Here's how the part is built. I have some questions about the finished solid (model axes, mm). Face numbers are marked on the shaded views. Round coordinates to 2 decimals unless told otherwise and drop trailing zeros. One line per item, written item: value. Start each with the question number.
Item 1: Thinking about a two-plate mould opening in Z: for the marked faces 1 and 2, which applies, released by +Z, released by -Z, zero draft, split by the parting line, or undercut?
Item 2: If I drill on line 1 (Y direction, x = -150.75, z = 1.25); line 2 (X direction, y = -2.25, z = 0.7); line 3 (X direction, y = 10.5, z = 0.45), over which ranges is the centre line in solid material (lowest first)?
Item 3: For P1, Ø8, axis at x = -150.75, y = 0, coming from the +Z side, with a flat end and sliding along its axis, tell me the tip position at first contact or that it passes through.
```python
from build123d import *

# Parameters (mm, degrees)
BOSS_EXTRUDE1_DEPTH = 3
SKETCH2_R           = 2.5
CUT_EXTRUDE1_DEPTH  = 4


with BuildPart() as part:
    # Sketch1 → Boss-Extrude1 (new body)
    with BuildSketch(Plane.XY):
        with BuildLine():
            Line((155.75, 15), (0, 15))
            Line((0, 15), (0, 0))
            Line((0, 0), (160.75, 0))
            Line((160.75, 0), (160.75, 10))
            ThreePointArc((160.75, 10), (159.285533906, 13.535533906), (155.75, 15))
        make_face()
        with BuildLine():
            Line((0, 15), (-155.75, 15))
            ThreePointArc((-155.75, 15), (-159.285533906, 13.535533906), (-160.75, 10))
            Line((-160.75, 10), (-160.75, 0))
            Line((-160.75, 0), (0, 0))
            Line((0, 0), (0, 15))
        make_face()
        with BuildLine():
            Line((0, -15), (0, 0))
            Line((0, 0), (-160.75, 0))
            Line((-160.75, 0), (-160.75, -10))
            ThreePointArc((-160.75, -10), (-159.285533906, -13.535533906), (-155.75, -15))
            Line((-155.75, -15), (0, -15))
        make_face()
        with BuildLine():
            Line((160.75, 0), (0, 0))
            Line((0, 0), (0, -15))
            Line((0, -15), (155.75, -15))
            ThreePointArc((155.75, -15), (159.285533906, -13.535533906), (160.75, -10))
            Line((160.75, -10), (160.75, 0))
        make_face()
    extrude(amount=BOSS_EXTRUDE1_DEPTH)

    # Sketch2 → Cut-Extrude1 (cut, through all)
    with BuildSketch(Plane(origin=(0, 0, 0), x_dir=(-1, 0, 0), z_dir=(0, 0, -1))):
        with BuildLine():
            ThreePointArc((-153.120541102, 0), (-150.620541102, -2.5), (-148.120541102, 0))
            Line((-148.120541102, 0), (-153.120541102, 0))
        make_face()
        with BuildLine():
            Line((-153.120541102, 0), (-148.120541102, 0))
            ThreePointArc((-148.120541102, 0), (-150.620541102, 2.5), (-153.120541102, 0))
        make_face()
        with Locations((150.75, 0)):
            Circle(SKETCH2_R)
    extrude(amount=-CUT_EXTRUDE1_DEPTH, mode=Mode.SUBTRACT)


solid = part.part
```
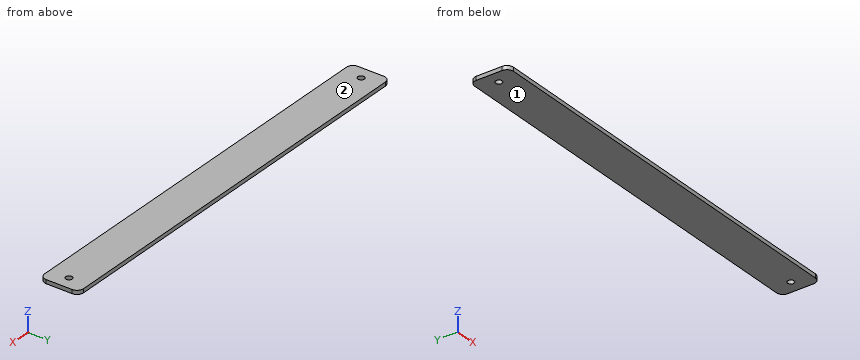
Values follow:
1. face 1: released by -Z
1. face 2: released by +Z
2. line 1: y = -15 to -2.5, 2.5 to 15
2. line 2: x = -160.75 to -151.84, -149.66 to 149.53, 151.71 to 160.75
2. line 3: x = -160.72 to 160.72
3. P1: stops at z = 3
